Autodesk Inventor part; units mm, degrees
ref_plane "YZ Plane" through (0, 0, 0) normal (1, 0, 0) x (0, 1, 0)
ref_plane "XZ Plane" through (0, 0, 0) normal (0, 1, 0) x (-1, 0, 0)
ref_plane "XY Plane" through (0, 0, 0) normal (0, 0, 1) x (1, 0, 0)
ref_plane "Arbeitsebene1" through (41.6445, -55.4632, -27.5498) normal (0, -1, 0) x (1, 0, 0)
sketch "Skizze1" plane through (41.6445, -55.4632, -27.5498) normal (0, -1, 0) x (1, 0, 0)
  line L0 (0, -17.58) -> (11, -17.58)
  line L1 (11, -17.58) -> (11, -68.08)
  line L2 (11, -68.08) -> (0, -68.08)
  line L3 (0, -68.08) -> (0, -17.58)
  line L4 (-20.1267, -68.08) -> (20.1267, -68.08)
  line L5 (0, 101.8556) -> (0, -98.0191)
  line L6 (0, -17.58) -> (-11, -17.58)
  line L7 (-11, -17.58) -> (-11, -68.08)
  line L8 (-11, -68.08) -> (0, -68.08)
  point P0 (-41.6445, 27.5498)
  dimension "d0" = 11
  dimension "d1" = 50.5
extrude "Extrusion1" add sketch "Skizze1" along normal blind 8
sketch "Skizze2" plane through (30.6445, -55.4632, -45.1298) normal (0, 0, 1) x (1, 0, 0)
  line L0 (22, 0) -> (0, 0)
  line L1 (0, 0) -> (0, -8)
  line L2 (22, -8) -> (0, -8)
  line L3 (22, 0) -> (22, -8)
  line L4 (21.5, -1.25) -> (0.5, -1.25)
  line L5 (0.5, -1.25) -> (0.5, -6.75)
  line L6 (0.5, -6.75) -> (21.5, -6.75)
  line L7 (21.5, -6.75) -> (21.5, -1.25)
  line L8 (21.5, -1.25) -> (0.5, -6.75) construction
  line L9 (0.5, -1.25) -> (21.5, -6.75) construction
  point P0 (-30.6445, 55.4632)
  point P1 (11, -4)
  dimension "d4" = 21
  dimension "d5" = 5.5
extrude "Extrusion2" cut sketch "Skizze2" against normal blind 17.5 contours L7 L6 L5 L4
properties part number "Außenhülle"
Model file for the job. Use its own axes, mm. A direction names the side the tool comes from. Round coordinates to 2 decimals unless told otherwise and drop trailing zeros. Write each loop counter-clockwise with the first axis right and the second up, starting at its lowest first coordinate (ties: lowest second). Pieces come first, ordered by that corner, then holes. Notation, with made-up numbers: (50.25, 24) -> (91.25, 24) arc R34 cw to (91.25, 60) -> close; hole circle Ø4 at (74, 69). An arc over 180 degrees is marked (long way). Answer as CSV lines item,"result".
1. Tool access for faces 1 (the face through (42, -56.713, -54)), 2 (the face through (42, -59, -95.63)): list every direction of +Z, -Z, +X, -X, +Y, -Y with a clear straight run to the whole face (end or side of a thin tool).
Resolved:
face 1,"+Z"
face 2,"-Z, +X, -X, +Y, -Y"
2. Drill centre lines: line 1 (X direction, y = -57.25, z = -56.5); line 2 (Y direction, x = 38.5, z = -56.5); line 3 (Z direction, x = 49.75, y = -58.75). Where is each one in solid material? Low to high.
Resolved:
line 1,"30.64 to 31.14, 52.14 to 52.64"
line 2,"-63.46 to -62.21, -56.71 to -55.46"
line 3,"-95.63 to -62.63"
3. Slice it at A-A, the plane z = -50. List the corners of the cut face in (x, y), plus the area to 3 significant figures.
Resolved:
outline,"(30.64, -63.46) -> (52.64, -63.46) -> (52.64, -55.46) -> (30.64, -55.46) -> close; hole (31.14, -62.21) -> (52.14, -62.21) -> (52.14, -56.71) -> (31.14, -56.71) -> close"
area,"60.5 mm²"
4. Slice it at B-B, the plane x = 43.5. List the corners of the cut face in (y, z).
Resolved:
outline,"(-63.46, -95.63) -> (-55.46, -95.63) -> (-55.46, -45.13) -> (-56.71, -45.13) -> (-56.71, -62.63) -> (-62.21, -62.63) -> (-62.21, -45.13) -> (-63.46, -45.13) -> close"
5. Pin check, flat tip, straight feed: pin 1 Ø1.6 at (x, y) = (43.5, -60) entering from +Z. Stop position of the tip, or through.
Resolved:
pin 1,"z = -62.63"
6. Slice it at C-C, the plane y = -58.75. List the corners of the cut face in (x, z).
Resolved:
outline,"(30.64, -95.63) -> (52.64, -95.63) -> (52.64, -45.13) -> (52.14, -45.13) -> (52.14, -62.63) -> (31.14, -62.63) -> (31.14, -45.13) -> (30.64, -45.13) -> close"
7. Mould opens along Y. For faces 3 (the face through (52.644, -59, -70)), 4 (the face through (41, -63.463, -70)), 5 (the face through (31.144, -59, -54)) say: +Y half, -Y half, draft (parallel to the pull), parting line (faces both ways), or undercut.
Resolved:
face 3,"draft"
face 4,"-Y half"
face 5,"undercut"
